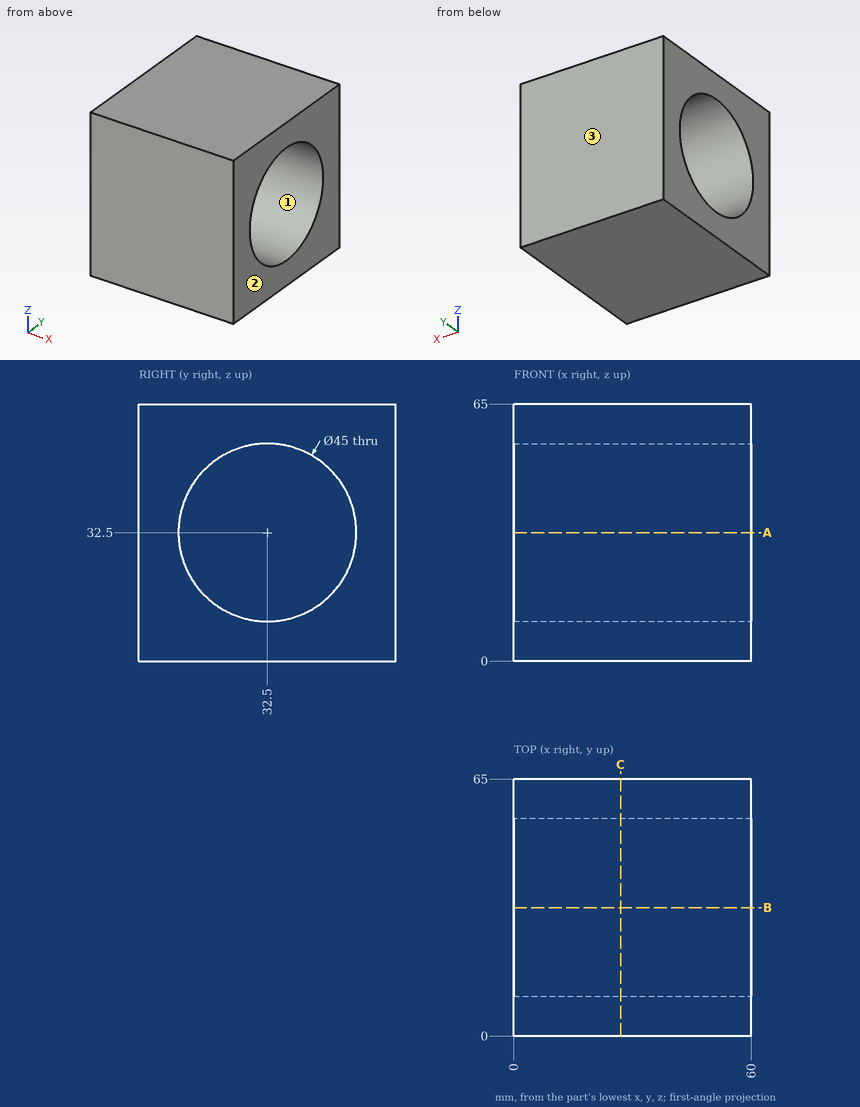
Input: dimensioned drawing with shaded views. Units: mm. Origin: part minimum x, y, z. Round coordinates to 2 decimals unless told otherwise and drop trailing zeros. Order: outer loops, then holes, each group sorted by start corner. A loop starts at its lowest first (then second) coordinate and runs counter-clockwise, first axis right, second up. Notation, with made-up numbers: (-1, -9) - (14, -9) arc R33 ccw to (14, 25) - close; hole circle Ø5 at (12.25, -34.75). An arc over 180 degrees is marked (long way). Use CSV: the item, a comma, the result in double quotes. Start each with the question number.
Q1. Mould query, pull axis Y, two halves, no side actions, for the marked faces 1, 2 and 3. Classes: +Y half, -Y half, draft (parallel to the pull), parting line (faces both ways), or undercut.
Q2. Material intervals for line 1 along Y through (x, z) = (40, 32); line 2 along Z through (x, y) = (14.5, 27.5), sorted ascending. Write a range as from..to.
Q3. Section query A-A (z = 32.5). Return loops of the section in (x, y), and give its area (3 significant figures).
Q4. Section query C-C (x = 27). Return loops of the section in (y, z).
Result set:
1,face 1,"undercut"
1,face 2,"draft"
1,face 3,"+Y half"
2,line 1,"y = 0..10.01, 54.99..65"
2,line 2,"z = 0..10.56, 54.44..65"
3,outline,"(0, 0) - (60, 0) - (60, 10) - (0, 10) - close; (0, 55) - (60, 55) - (60, 65) - (0, 65) - close"
3,area,"1,200 mm2"
4,outline,"(0, 0) - (65, 0) - (65, 65) - (0, 65) - close; hole circle Ø45 at (32.5, 32.5)"
